Geometry: final body of the model. Coordinates: model frame, mm. A direction names the side the tool comes from. Give positions to 0.01 mm unless a question says otherwise; leave off trailing zeros. Order: outer loops, then holes, each group sorted by start corner. A loop starts at its lowest first (then second) coordinate and runs counter-clockwise, first axis right, second up. Notation, with made-up numbers: (-25.75, 45.25) -> (13.25, 45.25) arc R26 cw to (13.25, 84.25) -> close; hole circle Ø7 at (29, -34.5). An arc over 180 degrees is marked (long way). One line per question, with ' | ' between items. Start each with the question number.
(1) Section A-A (z = -31). Return loops of the section in (x, y), then the cut area to 3 significant figures.
(2) Mould query, pull axis X, two halves, no side actions, for faces 4 (the face through (-118, 23, -27.94)), 5 (the face through (-118, 20.895, -19)), 6 (the face through (-137.082, 22, -7)). Classes: +X half, -X half, draft (parallel to the pull), parting line (faces both ways), or undercut.
(3) Section B-B (x = -128.5). Return loops of the section in (y, z).
(4) Set-up query: faces 1 (the face through (-118, 3, 0)), 2 (the face through (-98.982, 22, -7)), 3 (the face through (-118, 23, -33.02)). Return all of +Z, -Z, +X, -X, +Y, -Y with unobstructed straight access to the full face (end or side cutting, diameter ignored); none if empty.
(5) Section D-D (z = -8). Return loops of the section in (x, y).
(6) Ray query, L1, parallel to Y at x = -117, z = -22; L2, parallel to Z at x = -102, y = 5; L3, parallel to X at y = 21.5, z = -29. Return the intervals inside material, ascending.
(7) Section C-C (y = 2). Return loops of the section in (x, z).
(8) First-contact query: pin 1 Ø10 at (x, y) = (-107.5, 15) entering from -Z; pin 2 Ø12 at (x, z) = (-120, -14.5) entering from -Y. Flat tips, straight axial feed; report the tip coordinate or a pass-through.
```python
from build123d import *

# Parameters (mm, degrees)
SKETCH1_W           = 38.1
SKETCH1_H           = 35.56
BOSS_EXTRUDE1_DEPTH = 5.08
SKETCH2_W           = 38.1
SKETCH2_H           = 43.18
BOSS_EXTRUDE2_DEPTH = 5.08
CAVITY2_START       = -133.272192899
CAVITY2_OUTLINE_W   = 5.08
CAVITY2_OUTLINE_H   = 5.08
CAVITY2_DEPTH       = 30.48


# Read off the part's stored shape, not the designer's step: Cavity2
with BuildPart() as part:
    # Sketch1 → Boss-Extrude1 (new body)
    with BuildSketch(Plane.XY):
        with Locations((-118.032192899, 3.115408086)):
            Rectangle(SKETCH1_W, SKETCH1_H)
    extrude(amount=BOSS_EXTRUDE1_DEPTH)

    # Sketch2 → Boss-Extrude2 (add)
    with BuildSketch(Plane(origin=(0, 20.895408086, 0), x_dir=(1, 0, 0), z_dir=(0, 1, 0))):
        with Locations((-118.032192899, 16.51)):
            Rectangle(SKETCH2_W, SKETCH2_H)
    extrude(amount=BOSS_EXTRUDE2_DEPTH)

    # Cavity2 outline → Cavity2 (cut)
    with BuildSketch(Plane.YZ.offset(CAVITY2_START)):
        with Locations((23.435408086, -30.48)):
            Rectangle(CAVITY2_OUTLINE_W, CAVITY2_OUTLINE_H)
    extrude(amount=CAVITY2_DEPTH, mode=Mode.SUBTRACT)


solid = part.part
```
Response:
1) outline: (-137.08, 20.9) -> (-133.27, 20.9) -> (-133.27, 25.98) -> (-137.08, 25.98) -> close; (-102.79, 20.9) -> (-98.98, 20.9) -> (-98.98, 25.98) -> (-102.79, 25.98) -> close | area: 38.7 mm^2
2) face 4: undercut | face 5: draft | face 6: -X half
3) outline: (-14.66, 0) -> (20.9, 0) -> (20.9, -27.94) -> (25.98, -27.94) -> (25.98, 5.08) -> (-14.66, 5.08) -> close; (20.9, -38.1) -> (25.98, -38.1) -> (25.98, -33.02) -> (20.9, -33.02) -> close
4) face 1: -Z, +X, -X, -Y | face 2: +Z, -Z, +X, +Y, -Y | face 3: +Y, -Y
5) outline: (-137.08, 20.9) -> (-98.98, 20.9) -> (-98.98, 25.98) -> (-137.08, 25.98) -> close
6) L1: y = 20.9 to 25.98 | L2: z = 0 to 5.08 | L3: x = -137.08 to -133.27, -102.79 to -98.98
7) outline: (-137.08, 0) -> (-98.98, 0) -> (-98.98, 5.08) -> (-137.08, 5.08) -> close
8) pin 1: stops at z = 0 | pin 2: stops at y = 20.9
